from build123d import *

# Parameters (mm, degrees)
F0_W     = 29
F0_H     = 20
F0_R     = 1.25
F0_R_2   = 2
F1_DEPTH = 10
F2_DEPTH = 5
F3_DEPTH = 1
F4_DEPTH = 8
F5_DEPTH = 4
F6_R     = 4
F6_R_2   = 2
F7_DEPTH = 1
F8_SIZE  = 1.5


# Not quite as in the source:
# - a feature names something its author has since deleted; it is built from what else it names


with BuildPart() as f1:
    # F0 (on Top) → F1 (new body)
    with BuildSketch(Plane.XY):
        with Locations((14.5, -10)):
            Rectangle(F0_W, F0_H)
        with Locations((3, -17)):
            Circle(F0_R, mode=Mode.SUBTRACT)
        with Locations((26, -17)):
            Circle(F0_R, mode=Mode.SUBTRACT)
        with Locations((3, -3)):
            Circle(F0_R, mode=Mode.SUBTRACT)
        with BuildLine():
            Line((19, -17.75), (10, -17.75))
            ThreePointArc((10, -17.75), (2.25, -10), (10, -2.25))
            Line((10, -2.25), (19, -2.25))
            ThreePointArc((19, -2.25), (26.75, -10), (19, -17.75))
        make_face(mode=Mode.SUBTRACT)
        with Locations((26, -3)):
            Circle(F0_R, mode=Mode.SUBTRACT)
        with BuildLine():
            ThreePointArc((10, -2.25), (2.25, -10), (10, -17.75))
            Line((10, -17.75), (19, -17.75))
            ThreePointArc((19, -17.75), (26.75, -10), (19, -2.25))
            Line((19, -2.25), (10, -2.25))
        make_face()
        with BuildLine():
            ThreePointArc((10, -16.25), (3.75, -10), (10, -3.75))
            Line((10, -3.75), (19, -3.75))
            ThreePointArc((19, -3.75), (25.25, -10), (19, -16.25))
            Line((19, -16.25), (10, -16.25))
        make_face(mode=Mode.SUBTRACT)
        with BuildLine():
            Line((19, -3.75), (10, -3.75))
            ThreePointArc((10, -3.75), (3.75, -10), (10, -16.25))
            Line((10, -16.25), (19, -16.25))
            ThreePointArc((19, -16.25), (25.25, -10), (19, -3.75))
        make_face()
        with BuildLine():
            ThreePointArc((16.7443308628, -5.25927677), (24.25, -10), (16.7443308628, -14.74072323))
            ThreePointArc((16.7443308628, -14.74072323), (14.5, -15.75), (12.2556691372, -14.74072323))
            ThreePointArc((12.2556691372, -14.74072323), (4.75, -10), (12.2556691372, -5.25927677))
            ThreePointArc((12.2556691372, -5.25927677), (14.5, -4.25), (16.7443308628, -5.25927677))
        make_face(mode=Mode.SUBTRACT)
        with BuildLine():
            ThreePointArc((12.2556691372, -14.74072323), (14.5, -15.75), (16.7443308628, -14.74072323))
            ThreePointArc((16.7443308628, -14.74072323), (24.25, -10), (16.7443308628, -5.25927677))
            ThreePointArc((16.7443308628, -5.25927677), (14.5, -4.25), (12.2556691372, -5.25927677))
            ThreePointArc((12.2556691372, -5.25927677), (4.75, -10), (12.2556691372, -14.74072323))
        make_face()
        with Locations((10, -10)):
            Circle(F0_R_2, mode=Mode.SUBTRACT)
        with Locations((19, -10)):
            Circle(F0_R_2, mode=Mode.SUBTRACT)
        with Locations((19, -10)):
            Circle(F0_R_2)
        with Locations((3, -17)):
            Circle(F0_R)
        with Locations((26, -3)):
            Circle(F0_R)
    extrude(amount=-F1_DEPTH)

    # F0 (on Top) → F2 (cut)
    with BuildSketch(Plane.XY):
        with Locations((3, -3)):
            Circle(F0_R)
        with Locations((26, -3)):
            Circle(F0_R)
        with Locations((26, -17)):
            Circle(F0_R)
        with Locations((3, -17)):
            Circle(F0_R)
    extrude(amount=-F2_DEPTH, mode=Mode.SUBTRACT)

    # F0 (on Top) → F3 (cut)
    with BuildSketch(Plane.XY):
        with BuildLine():
            ThreePointArc((10, -2.25), (2.25, -10), (10, -17.75))
            Line((10, -17.75), (19, -17.75))
            ThreePointArc((19, -17.75), (26.75, -10), (19, -2.25))
            Line((19, -2.25), (10, -2.25))
        make_face()
        with BuildLine():
            ThreePointArc((10, -16.25), (3.75, -10), (10, -3.75))
            Line((10, -3.75), (19, -3.75))
            ThreePointArc((19, -3.75), (25.25, -10), (19, -16.25))
            Line((19, -16.25), (10, -16.25))
        make_face(mode=Mode.SUBTRACT)
    extrude(amount=-F3_DEPTH, mode=Mode.SUBTRACT)

    # F0 (on Top) → F4 (cut)
    with BuildSketch(Plane.XY):
        with Locations((19, -10)):
            Circle(F0_R_2)
    extrude(amount=-F4_DEPTH, mode=Mode.SUBTRACT)

    # F0 (on Top) → F5 (cut)
    with BuildSketch(Plane.XY):
        with BuildLine():
            ThreePointArc((12.2556691372, -14.74072323), (14.5, -15.75), (16.7443308628, -14.74072323))
            ThreePointArc((16.7443308628, -14.74072323), (24.25, -10), (16.7443308628, -5.25927677))
            ThreePointArc((16.7443308628, -5.25927677), (14.5, -4.25), (12.2556691372, -5.25927677))
            ThreePointArc((12.2556691372, -5.25927677), (4.75, -10), (12.2556691372, -14.74072323))
        make_face()
        with Locations((10, -10)):
            Circle(F0_R_2, mode=Mode.SUBTRACT)
        with Locations((19, -10)):
            Circle(F0_R_2, mode=Mode.SUBTRACT)
    extrude(amount=-F5_DEPTH, mode=Mode.SUBTRACT)

    # F6 (on face) → F7 (cut)
    with BuildSketch(Plane(origin=(0, 0, -10), x_dir=(1, 0, 0), z_dir=(0, 0, -1))):
        with Locations((10, 10)):
            Circle(F6_R)
        with Locations((10, 10)):
            Circle(F6_R_2, mode=Mode.SUBTRACT)
    extrude(amount=-F7_DEPTH, mode=Mode.SUBTRACT)

    # F8
    f8_edges = [f1.edges().sort_by_distance(p)[0] for p in [
        (29, -20, -5),
        (0, -20, -5),
        (0, 0, -5),
        (29, 0, -5),
    ]]
    chamfer(f8_edges, length=F8_SIZE)


solid = f1.part
The model under review builds one solid part; all positions refer to its coordinate system, in mm. A direction names the side the tool comes from. Round coordinates to 2 decimals unless told otherwise and drop trailing zeros. Loops run counter-clockwise (first coordinate to the right, second up) from the corner with the lowest first, then second, coordinate; pieces in that order, holes last. Notation, with made-up numbers: M -32,-17.5 L -13,-17.5 A31 cw -13,6.5 Z; hole C -25.5,47.5 d4. An arc over 180 degrees is marked long. Answer as CSV lines item,"result".
1. We need section A-A (z = -4.5). Give the boundary of the cut face in (x, y), plus the area to 3 significant figures.
Outcome:
outline,"M 0,-18.5 L 1.5,-20 L 27.5,-20 L 29,-18.5 L 29,-1.5 L 27.5,0 L 1.5,0 L 0,-1.5 Z; hole C 3,-17 d2.5; hole C 3,-3 d2.5; hole C 10,-10 d4; hole C 19,-10 d4; hole C 26,-17 d2.5; hole C 26,-3 d2.5"
area,"531 mm2"
2. Draft analysis for pull direction Y (two halves, no side actions). For faces 4 (the face through (16.8, -15.1, 0)), 5 (the face through (0.8, -0.7, -4.9)), 6 (the face through (14, -10, -4)), state which applies: pulls with the +Y half, pulls with the -Y half, needs draft (parallel to the pull), parting line crosses it, or undercut.
Outcome:
face 4,"needs draft"
face 5,"pulls with the +Y half"
face 6,"undercut"
3. We need section D-D (x = 3). Give the boundary of the cut face in (y, z), plus the area to 3 significant figures.
Outcome:
outline,"M -20,-10 L -4.25,-10 L -4.25,0 L -6.67,0 L -6.67,-1 L -13.33,-1 L -13.33,0 L -15.75,0 L -15.75,-5 L -18.25,-5 L -18.25,0 L -20,0 Z; M -1.75,-10 L 0,-10 L 0,0 L -1.75,0 Z"
area,"156 mm2"
4. We need section B-B (y = -10). Give the boundary of the cut face in (x, z).
Outcome:
outline,"M 0,-10 L 6,-10 L 6,-9 L 8,-9 L 8,-4 L 4.75,-4 L 4.75,0 L 3.75,0 L 3.75,-1 L 2.25,-1 L 2.25,0 L 0,0 Z; M 12,-9 L 14,-9 L 14,-10 L 29,-10 L 29,0 L 26.75,0 L 26.75,-1 L 25.25,-1 L 25.25,0 L 24.25,0 L 24.25,-4 L 21,-4 L 21,-8 L 17,-8 L 17,-4 L 12,-4 Z"
5. We need section C-C (x = 10.75). Give the boundary of the cut face in (y, z).
Outcome:
outline,"M -20,-10 L -13.93,-10 L -13.93,-9 L -11.85,-9 L -11.85,-4 L -15.2,-4 L -15.2,0 L -16.25,0 L -16.25,-1 L -17.75,-1 L -17.75,0 L -20,0 Z; M -8.15,-9 L -6.07,-9 L -6.07,-10 L 0,-10 L 0,0 L -2.25,0 L -2.25,-1 L -3.75,-1 L -3.75,0 L -4.8,0 L -4.8,-4 L -8.15,-4 Z"
6. To check wall thickness, follow L1, parallel to Y at x = 19, z = -2.7; L2, parallel to Y at x = 19, z = -6.35; L3, parallel to Y at x = 26, z = -2.85. State the ranges of each line that lie inside material, in increasing order. Write a range as [from, to].
Outcome:
L1,"y = [-20, -15.25], [-4.75, 0]"
L2,"y = [-20, -12], [-8, 0]"
L3,"y = [-20, -18.25], [-15.75, -4.25], [-1.75, 0]"
7. For faces 1 (the face through (3.75, -10.14, -0.49)), 2 (the face through (26.672, -15.946, -4.93)), 3 (the face through (6.004, -10.176, -9.507)), list the 3-axis set-ups (+Z, -Z, +X, -X, +Y, -Y) from which the entire face can be reached by the end or side of a thin tool; tool diameter is ignored.
Outcome:
face 1,"+Z"
face 2,"+Z, -Z"
face 3,"-Z"
8. Insertion check: pin 1 Ø3 at (x, y) = (26, -3.5) entering from +Z; pin 2 Ø4.5 at (x, y) = (10, -10) entering from -Z; pin 3 Ø1.2 at (x, y) = (19.5, -10) entering from +Z. Each pin has a flat end and moves straight along its axis. Give the tip position at first contact, or say it passes through.
Outcome:
pin 1,"stops at z = 0"
pin 2,"stops at z = -9"
pin 3,"stops at z = -8"
